CAD build for the part. Positions are in the model's coordinates, mm. Face numbers are marked on the shaded views. A direction names the side the tool comes from. Round coordinates to 2 decimals unless told otherwise and drop trailing zeros. Loops run counter-clockwise (first coordinate to the right, second up) from the corner with the lowest first, then second, coordinate; pieces in that order, holes last.
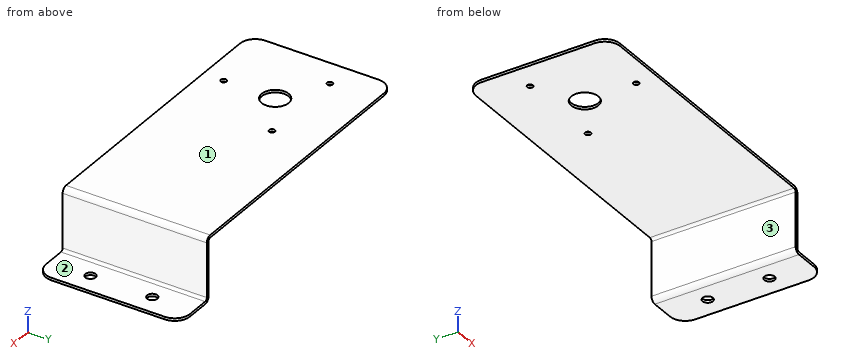
from build123d import *

# Parameters (mm, degrees)
F1_DEPTH = 44.45
F2_R     = 8.334375
F2_R_2   = 3.175
F2_R_3   = 1.7526
F3_DEPTH = 39.6885
F4_R     = 9.525


with BuildPart() as f1:
    # F0 (on Front) → F1 (new body, symmetric)
    with BuildSketch(Plane.XZ):
        with BuildLine():
            Line((-176.2125, 0), (-1.5875, 0))
            ThreePointArc((-1.5875, 0), (-0.464968, -0.464968), (0, -1.5875))
            Line((0, -1.5875), (0, -34.925))
            ThreePointArc((0, -34.925), (0.929936, -37.170064), (3.175, -38.1))
            Line((3.175, -38.1), (26.9875, -38.1))
            Line((26.9875, -38.1), (26.9875, -36.5125))
            Line((26.9875, -36.5125), (3.175, -36.5125))
            ThreePointArc((3.175, -36.5125), (2.052468, -36.047532), (1.5875, -34.925))
            Line((1.5875, -34.925), (1.5875, -1.5875))
            ThreePointArc((1.5875, -1.5875), (0.657564, 0.657564), (-1.5875, 1.5875))
            Line((-1.5875, 1.5875), (-176.2125, 1.5875))
            Line((-176.2125, 1.5875), (-176.2125, 0))
        make_face()
    extrude(amount=F1_DEPTH, both=True)

    # F2 (on face) → F3 (cut, through all)
    with BuildSketch(Plane.XY.offset(1.5875)):
        with Locations((-131.7625, 0)):
            Circle(F2_R)
        with Locations((14.2875, 19.05)):
            Circle(F2_R_2)
        with Locations((14.2875, -19.05)):
            Circle(F2_R_2)
        with Locations((-131.7625, -31.75)):
            Circle(F2_R_3)
        with Locations((-104.266193, 15.875)):
            Circle(F2_R_3)
        with Locations((-159.258807, 15.875)):
            Circle(F2_R_3)
    extrude(amount=-F3_DEPTH, mode=Mode.SUBTRACT)

    # F4
    f4_edges = [f1.edges().sort_by_distance(p)[0] for p in [
        (-176.2125, -44.45, 0.79375),
        (-176.2125, 44.45, 0.79375),
        (26.9875, 44.45, -37.30625),
        (26.9875, -44.45, -37.30625),
    ]]
    fillet(f4_edges, radius=F4_R)


solid = f1.part
Item 1: Wall check: L1, parallel to X at y = -25.5, z = -23; L2, parallel to Z at x = 11, y = 16.5. Give the ranges that are in metal, low to high.
Verdict:
L1: x = 0 to 1.59
L2: z = -38.1 to -36.51
Item 2: 3-axis set-ups, long thin cutter, end or side, ignore diameter. For the marked faces 1, 2 and 3: which of +Z, -Z, +X, -X, +Y, -Y reach the whole face in a straight line?
Verdict:
face 1: +Z, +X, -X, +Y, -Y
face 2: +Z, +X, +Y, -Y
face 3: -Z, -X, +Y, -Y
Item 3: Cut at C-C (z = -13.5). List the corners of the cut face in (x, y).
Verdict:
outline: (0, -44.45) - (1.59, -44.45) - (1.59, 44.45) - (0, 44.45) - close
Item 4: Flat gauge pins, fed straight in: P1, Ø4, axis at x = -131.76, y = -31.75, coming from the -Z side; P2, Ø10, axis at y = 16.5, z = -16.5, coming from the +X side; P3, Ø5.5, axis at x = 14.29, y = -19.05, coming from the -Z side (3 decimals); P4, Ø19, axis at x = 16, y = 0.5, coming from the +Z side. Where does each tip first touch, or does it go through?
Verdict:
P1: stops at z = 0
P2: stops at x = 1.59
P3: passes through
P4: stops at z = -36.51
Item 5: Cut at B-B (x = -73). List the corners of the cut face in (y, z).
Verdict:
outline: (-44.45, 0) - (44.45, 0) - (44.45, 1.59) - (-44.45, 1.59) - close
